from build123d import *

# Parameters (mm, degrees)
SKETCH1_W           = 25.4
SKETCH1_H           = 76.2
BOSS_EXTRUDE1_DEPTH = 25.4
SKETCH2_R           = 3.175
CUT_EXTRUDE1_DEPTH  = 96.038097624
SKETCH3_W           = 20.32
SKETCH3_H           = 45.72
CUT_EXTRUDE2_DEPTH  = 73.66
SKETCH4_R           = 6.35
BOSS_EXTRUDE2_DEPTH = 25.4


with BuildPart() as part:
    # Sketch1 → Boss-Extrude1 (new, symmetric)
    with BuildSketch(Plane.XY):
        with Locations((12.7, 38.1)):
            Rectangle(SKETCH1_W, SKETCH1_H)
    extrude(amount=BOSS_EXTRUDE1_DEPTH, both=True)

    # Sketch2 → Cut-Extrude1 (cut, through all)
    with BuildSketch(Plane.XY.offset(25.4)):
        with Locations((12.7, 38.1)):
            Circle(SKETCH2_R)
        with Locations((12.7, 63.5)):
            Circle(SKETCH2_R)
        with Locations((12.7, 88.9)):
            Circle(SKETCH2_R)
        with Locations((12.7, 12.7)):
            Circle(SKETCH2_R)
    extrude(amount=-CUT_EXTRUDE1_DEPTH, mode=Mode.SUBTRACT)

    # Sketch3 → Cut-Extrude2 (cut)
    with BuildSketch(Plane(origin=(0, 76.2, 0), x_dir=(1, 0, 0), z_dir=(0, 1, 0))):
        with Locations((12.7, 0)):
            Rectangle(SKETCH3_W, SKETCH3_H)
    extrude(amount=-CUT_EXTRUDE2_DEPTH, mode=Mode.SUBTRACT)

    # Sketch4 → Boss-Extrude2 (add)
    with BuildSketch(Plane.XZ):
        with Locations(Location((12.7, 0, 0), (0, 0, 270))):
            Circle(SKETCH4_R)
    extrude(amount=BOSS_EXTRUDE2_DEPTH)


solid = part.part
Design review of the part built by this model. Coordinates are the model's own, in mm. A direction names the side the tool comes from. Give positions to 0.01 mm unless a question says otherwise; leave off trailing zeros. Write each loop counter-clockwise with the first axis right and the second up, starting at its lowest first coordinate (ties: lowest second). Pieces come first, ordered by that corner, then holes. Notation, with made-up numbers: M -18.75,82 L 13.25,82 A17 cw 13.25,88 Z; hole C 54,84.25 d10. An arc over 180 degrees is marked long. Answer as a JSON object with one key per item and string values. Group by question number.
1) We need section C-C (z = 0). Give the boundary of the cut face in (x, y), and give its area (3 significant figures).
2) Tool access review of faces 5 (the face through (19, -12.5, 0.8)), 6 (the face through (2.54, 40, 0)), 7 (the face through (10.36, 65.646, 24.148)): name each direction out of +Z, -Z, +X, -X, +Y, -Y from which nothing blocks a thin tool from reaching the whole face with its end or side.
3) We need section D-D (x = 12.7). Count the separate pieces of the cut face and the enclosed holes in it, and give its area (3 significant figures).
4) Mouldability with a two-part tool opening along Y and no side actions: class faces 1 (the face through (2, 76.2, 2)), 2 (the face through (15.3, 0, 6)), 3 (the face through (0, 38, 0)), 4 (the face through (10.18, 36.17, 24.15)) as released by +Y, released by -Y, zero draft, split by the parting line, or undercut.
5) For line 1 along X through (y, z) = (43.5, -0.5); line 2 along Z through (x, y) = (20.75, 12); line 3 along Y through (x, z) = (23, 11), list the stretches that pass through material, from the lowest coordinate up.
6) We need section B-B (x = 4.5). Give the boundary of the cut face in (y, z), and give its area (3 significant figures).
7) Clearance check with flat-ended pins moving along their axes: pin 1 Ø1.5 at (x, z) = (5, 10.5) entering from -Y; pin 2 Ø5 at (x, z) = (17, -19.5) entering from +Y; pin 3 Ø10 at (x, y) = (12.7, 12.7) entering from -Z. State where each tip first meets the part, or that it passes through.
8) We need section A-A (y = 38.1). Give the boundary of the cut face in (x, z) (3 decimals), and give its area (3 significant figures).
Answer key:
{
 "1": {"outline": "M 0,0 L 6.35,0 L 6.35,-25.4 L 19.05,-25.4 L 19.05,0 L 25.4,0 L 25.4,76.2 L 22.86,76.2 L 22.86,2.54 L 2.54,2.54 L 2.54,76.2 L 0,76.2 Z", "area": "761 mm²"},
 "2": {"face 5": "-Y", "face 6": "+Y", "face 7": "+Z, -Z"},
 "3": {"separate pieces": "7", "enclosed holes": "0", "area": "729 mm²"},
 "4": {"face 1": "released by +Y", "face 2": "released by -Y", "face 3": "zero draft", "face 4": "undercut"},
 "5": {"line 1": "x = 0 to 2.54, 22.86 to 25.4", "line 2": "z = -25.4 to -22.86, 22.86 to 25.4", "line 3": "y = 0 to 76.2"},
 "6": {"outline": "M 0,-25.4 L 76.2,-25.4 L 76.2,-22.86 L 2.54,-22.86 L 2.54,22.86 L 76.2,22.86 L 76.2,25.4 L 0,25.4 Z", "area": "503 mm²"},
 "7": {"pin 1": "stops at y = 0", "pin 2": "stops at y = 2.54", "pin 3": "stops at z = -25.4"},
 "8": {"outline": "M 0,-25.4 L 9.525,-25.4 L 9.525,-22.86 L 2.54,-22.86 L 2.54,22.86 L 9.525,22.86 L 9.525,25.4 L 0,25.4 Z; M 15.875,-25.4 L 25.4,-25.4 L 25.4,25.4 L 15.875,25.4 L 15.875,22.86 L 22.86,22.86 L 22.86,-22.86 L 15.875,-22.86 Z", "area": "329 mm²"}
}
